Model file for the job. Use its own axes, mm. A direction names the side the tool comes from. Round coordinates to 2 decimals unless told otherwise and drop trailing zeros. Loops run counter-clockwise (first coordinate to the right, second up) from the corner with the lowest first, then second, coordinate; pieces in that order, holes last. Notation, with made-up numbers: (50, -39) -> (74, -39) arc R12 cw to (74, -33) -> close; hole circle Ø11 at (89.25, 82.25). An arc over 180 degrees is marked (long way). Use a Markdown table: item, result.
from build123d import *

# Parameters (mm, degrees)
SKETCH2_R           = 6.35
BOSS_EXTRUDE1_DEPTH = 2.54
BOSS_EXTRUDE2_DEPTH = 304.8


with BuildPart() as part:
    # Sketch2 → Boss-Extrude1 (new body)
    with BuildSketch(Plane.XY):
        Polygon((0, 0), (355.6, 0), (355.6, -101.6), (199.80781759, -101.6), (88.9, -279.4), (0, -279.4), align=None)
        with Locations((49.038050814, -254)):
            Circle(SKETCH2_R, mode=Mode.SUBTRACT)
    boss_extrude1 = extrude(amount=BOSS_EXTRUDE1_DEPTH)

    # Sketch3 → Boss-Extrude2 (add)
    with BuildSketch(Plane.XY.offset(2.54)):
        Polygon((2.54, -279.4), (2.54, -276.86), (2.54, -2.54), (353.06, -2.54), (353.06, -99.06), (198.398569196, -99.06), (87.490751606, -276.86), (87.490751606, -279.4), (88.9, -279.4), (199.80781759, -101.6), (355.6, -101.6), (355.6, 0), (0, 0), (0, -279.4), align=None)
    extrude(amount=BOSS_EXTRUDE2_DEPTH)

    # Mirror1: Boss-Extrude1 across plane
    add(boss_extrude1.mirror(Plane.XY.offset(154.94)))


solid = part.part
Q1. Flat gauge pins, fed straight in: pin 1 (1 mm diameter, centred on x = 141, z = 223.5, fed in from -Y); pin 2 (10 mm diameter, centred on x = 49.04, y = -254, fed in from +Z); pin 3 (6 mm diameter, centred on x = 159, z = 162, fed in from -Y). Where does each tip first touch, or does it go through?
Results list:
| item | result |
|---|---|
| pin 1 | stops at y = -196.68 |
| pin 2 | passes through |
| pin 3 | stops at y = -171.83 |
Q2. Band-saw the part on D-D, the plane y = -254. Give the cut face in (x, z), plus the area to 3 significant figures.
Results list:
| item | result |
|---|---|
| outline | (0, 0) -> (42.69, 0) -> (42.69, 2.54) -> (2.54, 2.54) -> (2.54, 307.34) -> (42.69, 307.34) -> (42.69, 309.88) -> (0, 309.88) -> close; (55.39, 0) -> (104.74, 0) -> (104.74, 309.88) -> (55.39, 309.88) -> (55.39, 307.34) -> (101.75, 307.34) -> (101.75, 2.54) -> (55.39, 2.54) -> close |
| area | 2,150 mm² |
Q3. Tool access for faces 1 (the face through (141, -108, 307.34)), 2 (the face through (48.211, -247.704, 308.628)), 3 (the face through (2.54, -143, 153)), 4 (the face through (279, -101.6, 157)), 5 (the face through (355.6, -50, 157)): list every direction of +Z, -Z, +X, -X, +Y, -Y with a clear straight run to the whole face (end or side of a thin tool).
Results list:
| item | result |
|---|---|
| face 1 | none |
| face 2 | +Z, -Z |
| face 3 | -Y |
| face 4 | +Z, -Z, +X, -Y |
| face 5 | +Z, -Z, +X, +Y, -Y |
Q4. Pull direction Z, two halves, no side cores. Call faces 6 (the face through (141, -107, 0)), 7 (the face through (2, -279.4, 156)), 8 (the face through (175, -2.54, 153)): released by +Z, released by -Z, zero draft, split by the parting line, or undercut.
Results list:
| item | result |
|---|---|
| face 6 | released by -Z |
| face 7 | zero draft |
| face 8 | undercut |
Q5. Band-saw the part on C-C, the plane z = 255.5. Give the cut face in (x, y), plus the area to 3 significant figures.
Results list:
| item | result |
|---|---|
| outline | (0, -279.4) -> (2.54, -279.4) -> (2.54, -2.54) -> (353.06, -2.54) -> (353.06, -99.06) -> (198.4, -99.06) -> (87.49, -276.86) -> (87.49, -279.4) -> (88.9, -279.4) -> (199.81, -101.6) -> (355.6, -101.6) -> (355.6, 0) -> (0, 0) -> close |
| area | 2,780 mm² |
Q6. Band-saw the part on A-A, the plane x = 319.5. Give the cut face in (y, z).
Results list:
| item | result |
|---|---|
| outline | (-101.6, 0) -> (0, 0) -> (0, 309.88) -> (-101.6, 309.88) -> close; hole (-99.06, 2.54) -> (-2.54, 2.54) -> (-2.54, 307.34) -> (-99.06, 307.34) -> close |
Q7. Band-saw the part on B-B, the plane y = -58. Give the cut face in (x, z), plus the area to 3 significant figures.
Results list:
| item | result |
|---|---|
| outline | (0, 0) -> (355.6, 0) -> (355.6, 309.88) -> (0, 309.88) -> close; hole (2.54, 2.54) -> (353.06, 2.54) -> (353.06, 307.34) -> (2.54, 307.34) -> close |
| area | 3,350 mm² |
Q8. Drill centre lines: L1, parallel to Z at x = 173.5, y = -66; L2, parallel to Y at x = 301, z = 128; L3, parallel to X at y = -49, z = 66. Where is each one in solid material? Low to high. Write a range as from..to.
Results list:
| item | result |
|---|---|
| L1 | z = 0..2.54, 307.34..309.88 |
| L2 | y = -101.6..-99.06, -2.54..0 |
| L3 | x = 0..2.54, 353.06..355.6 |
